Design review of the part shown in the three views and the two pictorial views. Dimensions are in mm from the part's minimum x, y and z. A direction names the side the tool comes from. Round coordinates to 2 decimals unless told otherwise and drop trailing zeros. Order: outer loops, then holes, each group sorted by start corner. A loop starts at its lowest first (then second) coordinate and runs counter-clockwise, first axis right, second up. Notation, with made-up numbers: (48.25, 11) - (100.25, 11) arc R24 ccw to (100.25, 42) - close; hole circle Ø7 at (5.5, 15.25). An arc over 180 degrees is marked (long way). One line per item, written item: value.
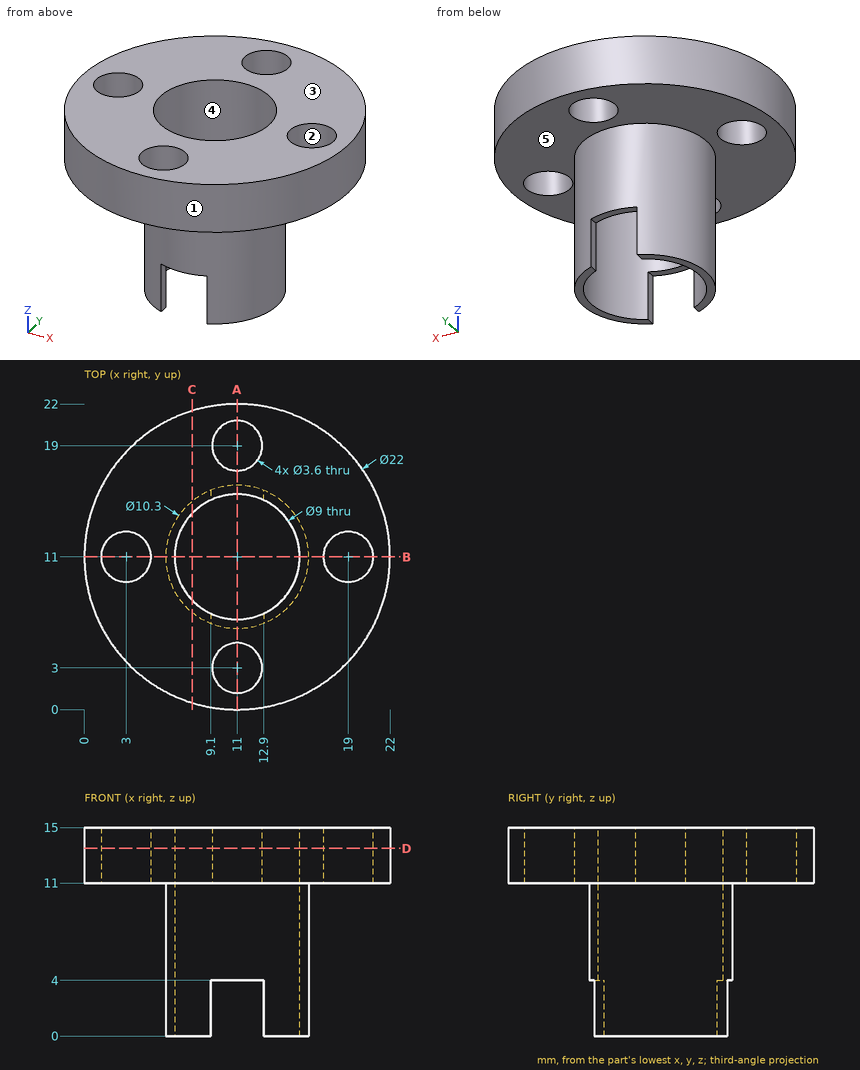
Item 1: Take a section at A-A (x = 11). Write out the cut boundary in (y, z), plus the area to 3 significant figures.
Returned:
outline: (0, 11) - (1.2, 11) - (1.2, 15) - (0, 15) - close; (4.8, 11) - (5.85, 11) - (5.85, 4) - (6.5, 4) - (6.5, 15) - (4.8, 15) - close; (15.5, 4) - (16.15, 4) - (16.15, 11) - (17.2, 11) - (17.2, 15) - (15.5, 15) - close; (20.8, 11) - (22, 11) - (22, 15) - (20.8, 15) - close
area: 32.3 mm^2
Item 2: Take a section at C-C (x = 7.75). Write out the cut boundary in (y, z) (3 decimals), plus the area to 3 significant figures.
Returned:
outline: (0.491, 11) - (7.005, 11) - (7.005, 0) - (7.888, 0) - (7.888, 15) - (0.491, 15) - close; (14.112, 0) - (14.995, 0) - (14.995, 11) - (21.509, 11) - (21.509, 15) - (14.112, 15) - close
area: 78.6 mm^2
Item 3: For P1, Ø0.8, axis at y = 6.5, z = 2, coming from the +X side; P2, Ø0.8, axis at y = 15.5, z = 1.5, coming from the -X side; P3, Ø6, axis at x = 19, y = 5.5, coming from the -Z side, all flat-tipped, find the tip position at first contact; note any pin that passes through.
Returned:
P1: x = 14.12
P2: x = 7.88
P3: z = 11
Item 4: Wall thickness on line 1 (Y direction, x = 11, z = 13.8); line 2 (X direction, y = 10.75, z = 9); line 3 (Y direction, x = 11, z = 9.5): over which ranges is each line inside the solid? List them lowest first.
Returned:
line 1: 0 to 1.2, 4.8 to 6.5, 15.5 to 17.2, 20.8 to 22
line 2: 5.86 to 6.51, 15.49 to 16.14
line 3: 5.85 to 6.5, 15.5 to 16.15
Item 5: Machinability: for the marked faces 4 and 5, which of the approach directions +Z, -Z, +X, -X, +Y, -Y give a long, thin tool a straight path to every point of the face, cutting with its end or side? Answer none if there is none.
Returned:
face 4: +Z, -Z
face 5: -Z
Item 6: The part is to be moulded in two halves that separate along Y. For the marked faces 1, 2 and 3, say which applies: +Y half, -Y half, draft (parallel to the pull), parting line (faces both ways), or undercut.
Returned:
face 1: parting line
face 2: undercut
face 3: draft
Item 7: Take a section at D-D (z = 13.5). Write out the cut boundary in (x, y), plus the area to 3 significant figures.
Returned:
outline: circle Ø22 at (11, 11); hole circle Ø3.6 at (3, 11); hole circle Ø9 at (11, 11); hole circle Ø3.6 at (11, 3); hole circle Ø3.6 at (11, 19); hole circle Ø3.6 at (19, 11)
area: 276 mm^2
Item 8: Take a section at B-B (y = 11). Write out the cut boundary in (x, z), plus the area to 3 significant figures.
Returned:
outline: (0, 11) - (1.2, 11) - (1.2, 15) - (0, 15) - close; (4.8, 11) - (5.85, 11) - (5.85, 0) - (6.5, 0) - (6.5, 15) - (4.8, 15) - close; (15.5, 0) - (16.15, 0) - (16.15, 11) - (17.2, 11) - (17.2, 15) - (15.5, 15) - close; (20.8, 11) - (22, 11) - (22, 15) - (20.8, 15) - close
area: 37.5 mm^2
